Geometry: final body of the model. Coordinates: model frame, mm. Face numbers are marked on the shaded views. A direction names the side the tool comes from. Round coordinates to 2 decimals unless told otherwise and drop trailing zeros. Write each loop counter-clockwise with the first axis right and the second up, starting at its lowest first coordinate (ties: lowest second). Pieces come first, ordered by that corner, then holes. Notation, with made-up numbers: M 18.5,16 L 55.5,16 A30 ccw 55.5,42 Z; hole C 84.25,28.5 d6. An arc over 180 degrees is marked long. Use one line per item in the form item = value. Start each with the question number.
Item 1: Ray query, probe 1 along X at (y, z) = (1.55, 0); probe 2 along X at (y, z) = (-16.5, -1); probe 3 along Y at (x, z) = (56, 3). Return the intervals inside material, ascending.
Item 2: Section query B-B (z = 0). Return loops of the section in (x, y), and give its area (3 significant figures).
Item 3: Pull-direction query (Y, two-part tool) for the marked faces 4, 5, 6 and 7; classes: pulls with the +Y half, pulls with the -Y half, needs draft (parallel to the pull), parting line crosses it, or undercut.
Item 4: Section query C-C (x = 15.5). Return loops of the section in (y, z).
Item 5: Section query A-A (y = -15). Return loops of the section in (x, z), and give its area (3 significant figures).
Item 6: Reachability of the marked faces 1, 2 and 3 from +Z, -Z, +X, -X, +Y, -Y: full face, straight path, thin tool, end or side. Return the list, or none.
Item 7: Section query D-D (x = 6). Return loops of the section in (y, z).
Item 8: Pin query (flat end, axial travel): pin 1 Ø2 at (x, z) = (69.5, -1.5) entering from -Y; pin 2 Ø4 at (y, z) = (-12, -2.5) entering from -X. Return the tip coordinate at first contact, or that it passes through.
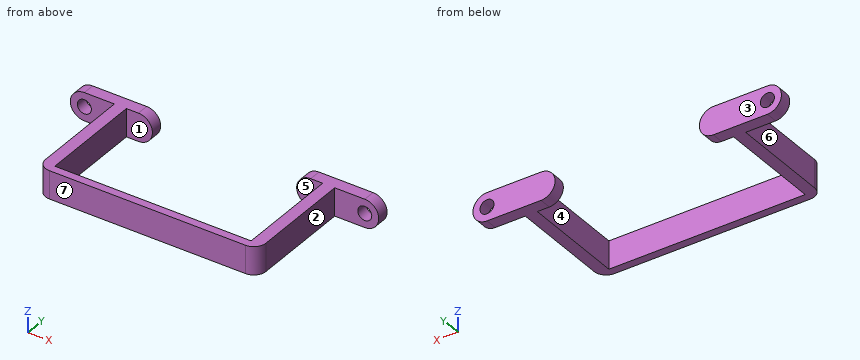
from build123d import *

# Parameters (mm, degrees)
SKETCH1_R           = 1.75
BOSS_EXTRUDE1_DEPTH = 3
SKETCH2_W           = 3
SKETCH2_H           = 7
BOSS_EXTRUDE2_DEPTH = 26
SKETCH3_W           = 27.49999964
SKETCH3_H           = 7
BOSS_EXTRUDE3_DEPTH = 2
FILLET1_R           = 3


with BuildPart() as part:
    # Sketch1 → Boss-Extrude1 (new body)
    with BuildSketch(Plane(origin=(0, 0, 0), x_dir=(1, 0, 0), z_dir=(0, 1, 0))):
        with BuildLine():
            Line((0, 3.5), (10.5, 3.5))
            Line((10.5, 3.5), (13.5, 3.5))
            ThreePointArc((13.5, 3.5), (17, 0), (13.5, -3.5))
            Line((13.5, -3.5), (10.5, -3.5))
            Line((10.5, -3.5), (0, -3.5))
            ThreePointArc((0, -3.5), (-3.5, 0), (0, 3.5))
        make_face()
        with Locations(Location((0, 0, 0), (0, 0, 270))):
            Circle(SKETCH1_R, mode=Mode.SUBTRACT)
    extrude(amount=BOSS_EXTRUDE1_DEPTH)

    # Sketch2 → Boss-Extrude2 (add)
    with BuildSketch(Plane(origin=(0, 0, 0), x_dir=(1, 0, 0), z_dir=(0, 1, 0))):
        with Locations((9, 0)):
            Rectangle(SKETCH2_W, SKETCH2_H)
    extrude(amount=-BOSS_EXTRUDE2_DEPTH)

    # Sketch3 → Boss-Extrude3 (add)
    with BuildSketch(Plane.XZ.offset(26)):
        with Locations((21.24999982, 0)):
            Rectangle(SKETCH3_W, SKETCH3_H)
    extrude(amount=BOSS_EXTRUDE3_DEPTH)

    # Fillet1
    fillet1_edges = [part.edges().sort_by_distance(p)[0] for p in [
        (7.5, -28, 0),
    ]]
    fillet(fillet1_edges, radius=FILLET1_R)

    # Mirror1: part across plane


with BuildPart() as part_1:
    add(part.part)
    add(part.part.mirror(Plane(origin=(34.99999964, -28, -3.5), x_dir=(0, 0, 1), z_dir=(-1, 0, 0))))


solid = part_1.part
Working result:
q1.probe_1 = -3.5 to -1.75, 1.75 to 17, 53 to 68.25, 71.75 to 73.5
q1.probe_2 = 7.5 to 10.5, 59.5 to 62.5
q1.probe_3 = -28 to -26, 0 to 3
q2.outline = M -3.5,0 L -1.75,0 L -1.75,3 L -3.5,3 Z; M 1.75,0 L 7.5,0 L 7.5,-25 A3 ccw 10.5,-28 L 59.5,-28 A3 ccw 62.5,-25 L 62.5,0 L 68.25,0 L 68.25,3 L 53,3 L 53,0 L 59.5,0 L 59.5,-26 L 10.5,-26 L 10.5,0 L 17,0 L 17,3 L 1.75,3 Z; M 71.75,0 L 73.5,0 L 73.5,3 L 71.75,3 Z
q2.area = 364 mm²
q3.face_4 = undercut
q3.face_5 = undercut
q3.face_6 = needs draft
q3.face_7 = pulls with the -Y half
q4.outline = M -28,-3.5 L -26,-3.5 L -26,3.5 L -28,3.5 Z; M 0,-2.87 L 3,-2.87 L 3,2.87 L 0,2.87 Z
q5.outline = M 7.5,-3.5 L 10.5,-3.5 L 10.5,3.5 L 7.5,3.5 Z; M 59.5,-3.5 L 62.5,-3.5 L 62.5,3.5 L 59.5,3.5 Z
q5.area = 42.0 mm²
q6.face_1 = +Z, -Z
q6.face_2 = +Z, -Z, +X, -Y
q6.face_3 = +Z, -Z, +X, -X, +Y
q7.outline = M 0,-3.5 L 3,-3.5 L 3,3.5 L 0,3.5 Z
q8.pin_1 = 0
q8.pin_2 = 7.5
